from build123d import *

# Parameters (mm, degrees)
F0_W     = 304.8
F0_H     = 38.1
F1_DEPTH = 12.7
F2_R     = 3.175
F3_DEPTH = 25.4
F4_R     = 3.175
F5_DEPTH = 25.4
F6_R     = 6.35
F7_DEPTH = 12.701


with BuildPart() as f1:
    # F0 (on Top) → F1 (new body)
    with BuildSketch(Plane.XY):
        with Locations((-152.4, 19.05)):
            Rectangle(F0_W, F0_H)
    extrude(amount=F1_DEPTH)

    # F2 (on face) → F3 (cut)
    with BuildSketch(Plane.YZ):
        with Locations((18.448802, 5.833903)):
            Circle(F2_R)
    extrude(amount=-F3_DEPTH, mode=Mode.SUBTRACT)

    # F4 (on face) → F5 (cut)
    with BuildSketch(Plane(origin=(-304.8, 0, 0), x_dir=(0, -1, 0), z_dir=(-1, 0, 0))):
        with Locations((-20.385453, 5.976154)):
            Circle(F4_R)
    extrude(amount=-F5_DEPTH, mode=Mode.SUBTRACT)

    # F6 (on face) → F7 (cut, through all)
    with BuildSketch(Plane.XY.offset(12.7)):
        with Locations((-247.65, 18.870285)):
            Circle(F6_R)
        with Locations((-57.15, 18.870285)):
            Circle(F6_R)
    extrude(amount=-F7_DEPTH, mode=Mode.SUBTRACT)


solid = f1.part
Could you check a few things on this model? Use its own coordinates, in mm. A direction names the side the tool comes from. Give positions to 0.01 mm unless a question says otherwise; leave off trailing zeros. Order: outer loops, then holes, each group sorted by start corner. A loop starts at its lowest first (then second) coordinate and runs counter-clockwise, first axis right, second up. Notation, with made-up numbers: (-19.75, 54) - (-14.75, 54) arc R4 ccw to (-14.75, 58) - close; hole circle Ø4 at (56.5, 17.25). An arc over 180 degrees is marked (long way). Return JSON: item names as keys, results as strings. Group by question number.
Q1. Please list where these lines run through material, in increasing order: line 1 along Y through (x, z) = (-57.15, 9); line 2 along X through (y, z) = (14, 8.5); line 3 along X through (y, z) = (21, 5.5). Write a range as [from, to].
Q2. Which directions (+Z, -Z, +X, -X, +Y, -Y) give clear straight access to the entire face, cutting with the end or side of a thin tool? Please do faces 4 (the face through (-12.522, 18.035, 8.982)), 5 (the face through (-279.4, 20, 6)), 6 (the face through (-155, 0, 6)).
Q3. Suppose I cut it at A-A, the plane x = -247.65. Please give me the cut outline in (y, z), and give its area (3 significant figures).
Q4. Thinking about a two-plate mould opening in Y: for faces 1 (the face through (-57.977, 25.166, 6.439)), 2 (the face through (-155, 38.1, 6)), 3 (the face through (0, 19, 10)), which applies, pulls with the +Y half, pulls with the -Y half, needs draft (parallel to the pull), parting line crosses it, or undercut?
Q5. Will this pin go through, and if not, where does the flat tip stop? pin 1 Ø7.5 at (x, y) = (-247.65, 18.87) entering from +Z.
Resolved:
{
 "1": {"line 1": "y = [0, 12.52], [25.22, 38.1]", "line 2": "x = [-304.8, -251.72], [-243.58, -61.22], [-53.08, 0]", "line 3": "x = [-279.4, -253.63], [-241.67, -63.13], [-51.17, -25.4]"},
 "2": {"face 4": "+X", "face 5": "-X", "face 6": "+Z, -Z, +X, -X, -Y"},
 "3": {"outline": "(0, 0) - (12.52, 0) - (12.52, 12.7) - (0, 12.7) - close; (25.22, 0) - (38.1, 0) - (38.1, 12.7) - (25.22, 12.7) - close", "area": "323 mm2"},
 "4": {"face 1": "undercut", "face 2": "pulls with the +Y half", "face 3": "needs draft"},
 "5": {"pin 1": "passes through"}
}
